Check sheet for the modelled part. Datum: model origin and axes. Units: mm. Face numbers are marked on the shaded views. A direction names the side the tool comes from. Coordinates: 2 decimals unless noted, no trailing zeros. Write each loop counter-clockwise with the first axis right and the second up, starting at its lowest first coordinate (ties: lowest second). Pieces come first, ordered by that corner, then holes. Notation, with made-up numbers: (-21, 32.5) -> (18, 32.5) arc R8 cw to (18, 36.5) -> close; hole circle Ø4 at (57, 86). An arc over 180 degrees is marked (long way). Put each result on its own line as item: value.
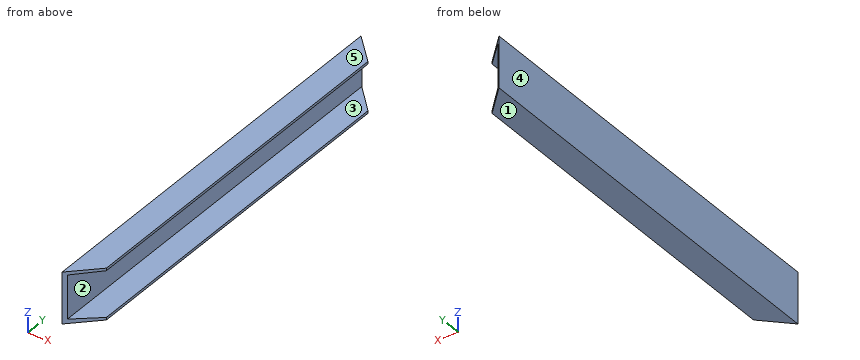
```python
from build123d import *

# Parameters (mm, degrees)
F1_DEPTH  = 800
F1_FACE_W = 50
F1_FACE_H = 800
F3_DEPTH  = 110


with BuildPart() as f1:
    # F0 (on Front) → F1 (new body)
    with BuildSketch(Plane.XZ):
        Polygon((0, 100), (0, 0), (50, 0), (50, 5), (6, 8.463486), (6, 93.463486), (50, 95), (50, 100), align=None)
    extrude(amount=F1_DEPTH)

    # F2 (on Top) + F1_face (on face) → F3 (cut)
    with BuildSketch(Plane.XY):
        Polygon((87.158154, 52.255962), (0, 52.255962), (0, 0), (87.158154, -87.158154), align=None)
        Polygon((0, -800), (0, -810), (98.867149, -810), (98.867149, -701.132851), align=None)
    with BuildSketch(Plane(origin=(25, -400, 100), x_dir=(1, 0, 0), z_dir=(0, 0, 1))):
        Rectangle(F1_FACE_W, F1_FACE_H)
    extrude(amount=F3_DEPTH, mode=Mode.SUBTRACT)


solid = f1.part
```
Q1. Material ranges on line 1 along X through (y, z) = (-342, 84); line 2 along Z through (x, y) = (38.5, -358); line 3 along Z through (x, y) = (24.5, -269), recorded low to high.
Recorded:
line 1: x = 0 to 6
line 2: z = 0 to 5.91, 94.6 to 100
line 3: z = 0 to 7.01, 94.11 to 100
Q2. Mould release check, pull along Z, two halves, no side actions. Record for the marked faces 3, 4 and 5: released by +Z, released by -Z, zero draft, split by the parting line, or undercut.
Recorded:
face 3: undercut
face 4: zero draft
face 5: released by +Z
Q3. Tool access check on the marked faces 1 and 2. Record the directions out of +Z, -Z, +X, -X, +Y, -Y that give a thin tool (end or side, any length) a straight path to the whole face; none if there is none.
Recorded:
face 1: -Z, +X, -X, +Y, -Y
face 2: +X, +Y, -Y
Q4. Depth check by flat-ended pin: P1, Ø10, axis at x = 14.5, z = 30.5, coming from the +Y side. Enter the tip coordinate at first touch or a pass-through.
Recorded:
P1: passes through
Q5. Cross-section at B-B (y = -489). Record the cut outline in (x, z).
Recorded:
outline: (0, 0) -> (50, 0) -> (50, 5) -> (6, 8.46) -> (6, 93.46) -> (50, 95) -> (50, 100) -> (0, 100) -> close
Q6. Cross-section at C-C (z = 41). Record the cut outline in (x, y).
Recorded:
outline: (0, -800) -> (6, -794) -> (6, -6) -> (0, 0) -> close
Q7. Cross-section at A-A (x = 25). Record the cut outline in (y, z), plus the area to 3 significant figures.
Recorded:
outline: (-775, 0) -> (-25, 0) -> (-25, 6.97) -> (-775, 6.97) -> close; (-775, 94.13) -> (-25, 94.13) -> (-25, 100) -> (-775, 100) -> close
area: 9,630 mm2
